from build123d import *

# Parameters (mm, degrees)
F1_DEPTH = 25.4


with BuildPart() as f1:
    # F0 (on Top) → F1 (new body)
    with BuildSketch(Plane.XY):
        with BuildLine():
            ThreePointArc((-44.240825, 0), (-59.249237, -15.008412), (-44.240825, -30.016825))
            Line((-44.240825, -30.016825), (-1.568824, -30.016825))
            Line((-1.568824, -30.016825), (40.475648, -30.016825))
            Line((40.475648, -30.016825), (41.103177, -30.016825))
            ThreePointArc((41.103177, -30.016825), (56.111589, -15.008412), (41.103177, 0))
            Line((41.103177, 0), (40.894002, 0))
            Line((40.894002, 0), (0, 0))
            Line((0, 0), (-1.568824, 0))
            Line((-1.568824, 0), (-44.240825, 0))
        make_face()
        Polygon((-44.240825, 18.930471), (-44.240825, 0), (-1.568824, 0), (0, 0), (40.894002, 0), (40.894002, 18.930471), align=None)
    extrude(amount=F1_DEPTH)


solid = f1.part
The model under review builds one solid part; all positions refer to its coordinate system, in mm. A direction names the side the tool comes from. Give positions to 0.01 mm unless a question says otherwise; leave off trailing zeros. Write each loop counter-clockwise with the first axis right and the second up, starting at its lowest first coordinate (ties: lowest second). Pieces come first, ordered by that corner, then holes. Notation, with made-up numbers: M 20.25,-2 L 73.25,-2 A21 ccw 73.25,31 Z; hole C 24,19.5 d5. An arc over 180 degrees is marked long. One line per question, with ' | ' between items. Start each with the question number.
Item 1: Wall thickness on line 1 (X direction, y = 5, z = 8.75); line 2 (Y direction, x = -53, z = 19); line 3 (X direction, y = -8.5, z = 8.5): over which ranges is each line inside the solid? List them lowest first. Write a range as from..to.
Item 2: For pin 1 (5.5 mm diameter, centred on y = 7, z = 14.5, fed in from +X); pin 2 (15 mm diameter, centred on y = 5, z = 14, fed in from -X); pin 3 (12 mm diameter, centred on y = -7.5, z = 13, fed in from -X), all flat-tipped, find the tip position at first contact; note any pin that passes through.
Item 3: We need section B-B on y = 9. Write out the cut boundary in (x, z).
Item 4: We need section C-C on y = -22.5. Write out the cut boundary in (x, z).
Item 5: We need section A-A on z = 5.75. Write out the cut boundary in (x, y), plus the area to 3 significant figures.
Item 6: For faces 1 (the flat face through (-44.241, 10, 13)), 2 (the flat face through (-2, -30.017, 13)), 3 (the flat face through (40.894, 9, 13)), list the 3-axis set-ups (+Z, -Z, +X, -X, +Y, -Y) from which the entire face can be reached by the end or side of a thin tool; tool diameter is ignored.
Results found:
1) line 1: x = -44.24..40.89 | line 2: y = -27.2..-2.82 | line 3: x = -57.76..54.63
2) pin 1: stops at x = 40.89 | pin 2: stops at x = -52.53 | pin 3: stops at x = -59.17
3) outline: M -44.24,0 L 40.89,0 L 40.89,25.4 L -44.24,25.4 Z
4) outline: M -57.25,0 L 54.11,0 L 54.11,25.4 L -57.25,25.4 Z
5) outline: M -44.24,-30.02 L 41.1,-30.02 A15.01 ccw 41.1,0 L 40.89,0 L 40.89,18.93 L -44.24,18.93 L -44.24,0 A15.01 ccw Z | area: 4,880 mm2
6) face 1: +Z, -Z, -X, +Y | face 2: +Z, -Z, +X, -X, -Y | face 3: +Z, -Z, +X, +Y
